The listing builds one solid part. Answer for the finished solid, in the listing's coordinates (mm). A direction names the side the tool comes from. Give positions to 0.01 mm unless a question says otherwise; leave off trailing zeros. Loops run counter-clockwise (first coordinate to the right, second up) from the corner with the lowest first, then second, coordinate; pieces in that order, holes last.
Item 1: A tool of negligible diameter and unlimited length cuts with its end or side. For faces 1 (the face through (31, 3, -49)), 2 (the face through (66, 3, -47.722)), 3 (the face through (66, 3.336, -24)), from which of +Z, -Z, +X, -X, +Y, -Y can it reach the whole face along a straight path? Write none if from no direction.
Item 2: Section A-A, the plane z = -24.5 is taken. Give the vertices of the cut face in (x, y).
Item 3: The mould has two halves that part along Y. Classify faces 4 (the face through (66, 1.909, -24)), 5 (the face through (66, 3, -1.278)), 6 (the face through (31, 5.8, -25)): pulls with the +Y half, pulls with the -Y half, needs draft (parallel to the pull), parting line crosses it, or undercut.
Item 4: Each of these flat-tipped pins is pushed along its axis until it touches: pin 1 Ø1.1 at (y, z) = (2.5, -31.5) entering from +X; pin 2 Ø3 at (x, z) = (67, -25.5) entering from +Y; pin 3 Ø1.1 at (x, y) = (66, 2.5) entering from -Z. Where does it stop, or does it pass through?
Item 5: Section B-B, the plane x = 64.5 is taken. Give the vertices of the cut face in (y, z), and give its area (3 significant figures).
Item 6: Consider line 1 along X through (y, z) = (3.65, -41); line 2 along X through (y, z) = (3.3, -3.5); line 3 along Y through (x, z) = (68.5, -43). Determine where each line is inside the solid, lowest interval first.
from build123d import *

# Parameters (mm, degrees)
CROQUIS1_W              = 63
CROQUIS1_H              = 49
SALIENTE_EXTRUIR1_DEPTH = 5.8
REDONDEO1_R             = 1.5
CROQUIS2_W              = 46.443628054
CROQUIS2_H              = 1.426596084
SALIENTE_EXTRUIR2_DEPTH = 6
CROQUIS3_R              = 0.510026017
CROQUIS3_R_2            = 0.496056104
SALIENTE_EXTRUIR3_DEPTH = 5


with BuildPart() as part:
    # Croquis1 → Saliente-Extruir1 (new body)
    with BuildSketch(Plane(origin=(0, 0, 0), x_dir=(1, 0, 0), z_dir=(0, 1, 0))):
        with Locations((31.5, 24.5)):
            Rectangle(CROQUIS1_W, CROQUIS1_H)
    extrude(amount=SALIENTE_EXTRUIR1_DEPTH)

    # Redondeo1
    redondeo1_edges = [part.edges().sort_by_distance(p)[0] for p in [
        (31.5, 5.8, -49),
        (31.5, 0, -49),
        (31.5, 0, 0),
        (31.5, 5.8, 0),
    ]]
    fillet(redondeo1_edges, radius=REDONDEO1_R)

    # Croquis2 → Saliente-Extruir2 (add)
    with BuildSketch(Plane(origin=(63, 0, 0), x_dir=(0, 0, -1), z_dir=(1, 0, 0))):
        with Locations((24.5, 2.622606317)):
            Rectangle(CROQUIS2_W, CROQUIS2_H)
    extrude(amount=SALIENTE_EXTRUIR2_DEPTH)

    # Croquis3 → Saliente-Extruir3 (add)
    with BuildSketch(Plane(origin=(69, 0, 0), x_dir=(0, 0, -1), z_dir=(1, 0, 0))):
        with Locations((21.5, 2.616385566)):
            Circle(CROQUIS3_R)
        with Locations((27.5, 2.616385566)):
            Circle(CROQUIS3_R_2)
    extrude(amount=SALIENTE_EXTRUIR3_DEPTH)


solid = part.part
Worked answers:
1. face 1: -Z, +X, -X, +Y, -Y
1. face 2: -Z, +X, +Y, -Y
1. face 3: +Z, -Z, +X, +Y
2. outline: (0, 0) - (63, 0) - (63, 1.91) - (69, 1.91) - (69, 3.34) - (63, 3.34) - (63, 5.8) - (0, 5.8) - close
3. face 4: pulls with the -Y half
3. face 5: needs draft
3. face 6: pulls with the +Y half
4. pin 1: stops at x = 69
4. pin 2: stops at y = 3.34
4. pin 3: stops at z = -47.72
5. outline: (1.91, -47.72) - (3.34, -47.72) - (3.34, -1.28) - (1.91, -1.28) - close
5. area: 66.3 mm2
6. line 1: x = 0 to 63
6. line 2: x = 0 to 69
6. line 3: y = 1.91 to 3.34
